from build123d import *

# Parameters (mm, degrees)
BOSS_EXTRUDE1_DEPTH = 4.7752
SKETCH1_3_R         = 1.5
CUT_EXTRUDE1_DEPTH  = 5.7752
CUT_EXTRUDE2_DEPTH  = 10


with BuildPart() as part:
    # Sketch1 → Boss-Extrude1 (new body)
    with BuildSketch(Plane.XY):
        with BuildLine():
            Line((0, 24.8876), (-4.7752, 24.8876))
            Line((-4.7752, 24.8876), (-4.7752, 40))
            ThreePointArc((-4.7752, 40), (-6.239666094, 43.535533906), (-9.7752, 45))
            Line((-9.7752, 45), (-49.7752, 45))
            ThreePointArc((-49.7752, 45), (-53.310733906, 43.535533906), (-54.7752, 40))
            Line((-54.7752, 40), (-54.7752, 24.8876))
            Line((-54.7752, 24.8876), (-59.5504, 24.8876))
            Line((-59.5504, 24.8876), (-59.5504, 42.5))
            Line((-59.5504, 42.5), (-69.5504, 42.5))
            Line((-69.5504, 42.5), (-69.5504, 2.5))
            Line((-69.5504, 2.5), (-59.5504, 2.5))
            Line((-59.5504, 2.5), (-59.5504, 20.1124))
            Line((-59.5504, 20.1124), (-54.7752, 20.1124))
            Line((-54.7752, 20.1124), (-54.7752, 5))
            ThreePointArc((-54.7752, 5), (-53.310733906, 1.464466094), (-49.7752, 0))
            Line((-49.7752, 0), (-9.7752, 0))
            ThreePointArc((-9.7752, 0), (-6.239666094, 1.464466094), (-4.7752, 5))
            Line((-4.7752, 5), (-4.7752, 20.1124))
            Line((-4.7752, 20.1124), (0, 20.1124))
            Line((0, 20.1124), (0, 2.5))
            Line((0, 2.5), (10, 2.5))
            Line((10, 2.5), (10, 42.5))
            Line((10, 42.5), (0, 42.5))
            Line((0, 42.5), (0, 24.8876))
        make_face()
    extrude(amount=BOSS_EXTRUDE1_DEPTH)

    # Sketch1_3 → Cut-Extrude1 (cut, through all)
    with BuildSketch(Plane.XY):
        with BuildLine():
            ThreePointArc((-63.0504, 37.5), (-64.5504, 36), (-66.0504, 37.5))
            Line((-66.0504, 37.5), (-66.0504, 7.5))
            ThreePointArc((-66.0504, 7.5), (-64.5504, 9), (-63.0504, 7.5))
            Line((-63.0504, 7.5), (-63.0504, 37.5))
        make_face()
        with Locations((-64.5504, 37.5)):
            Circle(SKETCH1_3_R)
        with Locations((-64.5504, 7.5)):
            Circle(SKETCH1_3_R)
        with BuildLine():
            ThreePointArc((6.5, 37.5), (5, 36), (3.5, 37.5))
            Line((3.5, 37.5), (3.5, 7.5))
            ThreePointArc((3.5, 7.5), (5, 9), (6.5, 7.5))
            Line((6.5, 7.5), (6.5, 37.5))
        make_face()
        with Locations((5, 7.5)):
            Circle(SKETCH1_3_R)
        with Locations((5, 37.5)):
            Circle(SKETCH1_3_R)
    extrude(amount=CUT_EXTRUDE1_DEPTH, mode=Mode.SUBTRACT)

    # Sketch1_5 → Cut-Extrude2 (cut)
    with BuildSketch(Plane.XY):
        with BuildLine():
            Line((-9.7752, 42), (-5.192624305, 42))
            ThreePointArc((-5.192624305, 42), (-7.036587212, 44.183300133), (-9.7752, 45))
            Line((-9.7752, 45), (-9.7752, 42))
        make_face()
        with BuildLine():
            Line((-54.357775695, 42), (-9.7752, 42))
            Line((-9.7752, 42), (-9.7752, 45))
            Line((-9.7752, 45), (-49.7752, 45))
            ThreePointArc((-49.7752, 45), (-52.513812788, 44.183300133), (-54.357775695, 42))
        make_face()
        with BuildLine():
            ThreePointArc((-9.7752, 0), (-7.036587212, 0.816699867), (-5.192624305, 3))
            Line((-5.192624305, 3), (-9.7752, 3))
            Line((-9.7752, 3), (-54.357775695, 3))
            ThreePointArc((-54.357775695, 3), (-52.513812788, 0.816699867), (-49.7752, 0))
            Line((-49.7752, 0), (-9.7752, 0))
        make_face()
    extrude(amount=CUT_EXTRUDE2_DEPTH, mode=Mode.SUBTRACT)


solid = part.part
Source: CAD feature listing. Evaluate the final solid. Frame: model axes, mm. A direction names the side the tool comes from. Give positions to 0.01 mm unless a question says otherwise; leave off trailing zeros. Write each loop counter-clockwise with the first axis right and the second up, starting at its lowest first coordinate (ties: lowest second). Pieces come first, ordered by that corner, then holes. Notation, with made-up numbers: (38.25, 82.25) - (54.25, 82.25) arc R17 cw to (54.25, 93.25) - close; hole circle Ø5 at (63.25, 81.25). An arc over 180 degrees is marked (long way). Write item = value, one per line. Start each with the question number.
Q1. Material intervals for probe 1 along X at (y, z) = (29, 2.8); probe 2 along X at (y, z) = (22, 2.3); probe 3 along X at (y, z) = (40, 0.7), sorted ascending.
Q2. Cut plane A-A, the plane y = 34.5. Return loops of the section in (x, z).
Q3. Cut plane C-C, the plane x = 5. Return loops of the section in (y, z), then the cut area to 3 significant figures.
Q4. Cut plane B-B, the plane z = 2.2. Give the number of separate pieces and of enclosed holes in the cut face, then the cut area to 3 significant figures.
Q5. Reachability of faces 1 (the cylindrical face through (-54.667, 41.036, 2.354)), 2 (the flat face through (5, 42.5, 2)), 3 (the flat face through (-2, 20.112, 2)), 4 (the flat face through (-66.05, 23, 2)) from +Z, -Z, +X, -X, +Y, -Y: full face, straight path, thin tool, end or side. Return the list, or none.
Q6. Draft query along X for faces 5 (the flat face through (-69.55, 23, 2)), 6 (the flat face through (-30, 42, 2)), 7 (the flat face through (-64, 42.5, 2)). Return one class per face: +X half, -X half, draft (parallel to the pull), parting line (faces both ways), or undercut.
Q7. Pin query (flat end, axial travel): pin 1 Ø10 at (x, y) = (-5, 15) entering from -Z; pin 2 Ø1.4 at (x, z) = (-56.5, 3.5) entering from -Y; pin 3 Ø1 at (x, z) = (-18.5, 2.5) entering from +Y; pin 4 Ø1.4 at (x, z) = (-57.5, 3.5) entering from +Y. Return the tip coordinate at first contact, or that it passes through.
Q8. Cut plane D-D, the plane y = 21.5. Return loops of the section in (x, z), then the cut area to 3 significant figures.
Computed values:
q1.probe_1 = -69.55 to -66.05, -63.05 to -59.55, -54.78 to -4.78, 0 to 3.5, 6.5 to 10
q1.probe_2 = -69.55 to -66.05, -63.05 to 3.5, 6.5 to 10
q1.probe_3 = -69.55 to -59.55, -54.78 to -4.78, 0 to 10
q2.outline = (-69.55, 0) - (-66.05, 0) - (-66.05, 4.78) - (-69.55, 4.78) - close; (-63.05, 0) - (-59.55, 0) - (-59.55, 4.78) - (-63.05, 4.78) - close; (-54.78, 0) - (-4.78, 0) - (-4.78, 4.78) - (-54.78, 4.78) - close; (0, 0) - (3.5, 0) - (3.5, 4.78) - (0, 4.78) - close; (6.5, 0) - (10, 0) - (10, 4.78) - (6.5, 4.78) - close
q3.outline = (2.5, 0) - (6, 0) - (6, 4.78) - (2.5, 4.78) - close; (39, 0) - (42.5, 0) - (42.5, 4.78) - (39, 4.78) - close
q3.area = 33.4 mm²
q4.separate_pieces = 1
q4.enclosed_holes = 2
q4.area = 2,600 mm²
q5.face_1 = +Z, -Z, +Y
q5.face_2 = +Z, -Z, +X, -X, +Y
q5.face_3 = +Z, -Z, -Y
q5.face_4 = +Z, -Z
q6.face_5 = -X half
q6.face_6 = undercut
q6.face_7 = draft
q7.pin_1 = 0
q7.pin_2 = 20.11
q7.pin_3 = 42
q7.pin_4 = 24.89
q8.outline = (-69.55, 0) - (-66.05, 0) - (-66.05, 4.78) - (-69.55, 4.78) - close; (-63.05, 0) - (3.5, 0) - (3.5, 4.78) - (-63.05, 4.78) - close; (6.5, 0) - (10, 0) - (10, 4.78) - (6.5, 4.78) - close
q8.area = 351 mm²
